```python
from build123d import *

# Parameters (mm, degrees)
F0_R      = 1.75
F0_R_2    = 1.51
F0_R_3    = 1.225
F8_DEPTH  = 0.5
F2_R      = 1.75
F2_R_2    = 1.51
F2_R_3    = 1.225
F9_DEPTH  = 0.5
F7_R      = 1.97
F10_DEPTH = 0.5
F11_DEPTH = 1
F12_DEPTH = 0.5
F13_DEPTH = 25
F16_DEPTH = 0.5
F17_DEPTH = 0.5
F18_W     = 41.976
F18_H     = 1.2
F19_DEPTH = 11.301


# Not quite as in the source:
# - a feature names something its author has since deleted; it is built from what else it names


with BuildPart() as f8:
    # F0 (on Front) → F8 (new body)
    with BuildSketch(Plane.XZ):
        with BuildLine():
            Line((-24.095, 11.6), (-47.125, 11.6))
            Line((-47.125, 11.6), (-47.125, 0))
            Line((-47.125, 0), (47.125, 0))
            ThreePointArc((47.125, 0), (48.3457892371, 4.0785044966), (44.6764603032, 6.2373353065))
            Line((44.6764603032, 6.2373353065), (25.9870177338, 8.0793821146))
            Line((25.9870177338, 8.0793821146), (-19.4229822662, 8.0793821146))
            Line((-19.4229822662, 8.0793821146), (-24.095, 11.6))
        make_face()
        with Locations((-43.275, 3.85)):
            Circle(F0_R, mode=Mode.SUBTRACT)
        with Locations((45.1343327214, 2.8178092836)):
            Circle(F0_R_2, mode=Mode.SUBTRACT)
        with Locations((-40.8, 8.615)):
            Circle(F0_R_3, mode=Mode.SUBTRACT)
    extrude(amount=F8_DEPTH)

    # F6 (on offset) → F9, piece 2 (join)
    with BuildSketch(Plane.YZ.offset(-47.125)):
        Polygon((3.7804580054, 10.7198863682), (3, 11.65), (0, 11.65), (0, 0), (4.5804580054, 0), (4.5804580054, 10.7198863682), align=None)
    extrude(amount=F9_DEPTH)



with BuildPart() as f8b:
    # F2 (on offset) → F8, piece 2 (new body)
    with BuildSketch(Plane.XZ.offset(-10.8)):
        with BuildLine():
            Line((-19.4229822662, 8.0793821146), (-24.095, 11.6))
            Line((-24.095, 11.6), (-47.125, 11.6))
            Line((-47.125, 11.6), (-47.125, 0))
            Line((-47.125, 0), (47.125, 0))
            ThreePointArc((47.125, 0), (48.3457892371, 4.0785044966), (44.6764603032, 6.2373353065))
            Line((44.6764603032, 6.2373353065), (25.9870177338, 8.0793821146))
            Line((25.9870177338, 8.0793821146), (-19.4229822662, 8.0793821146))
        make_face()
        with Locations((-43.275, 3.85)):
            Circle(F2_R, mode=Mode.SUBTRACT)
        with Locations((45.1343327214, 2.8178092836)):
            Circle(F2_R_2, mode=Mode.SUBTRACT)
        with Locations((-40.8, 8.615)):
            Circle(F2_R_3, mode=Mode.SUBTRACT)
    extrude(amount=F8_DEPTH)

    # F6 (on offset) → F9 (join)
    with BuildSketch(Plane.YZ.offset(-47.125)):
        Polygon((10.8, 0), (10.8, 11.65), (7.8, 11.65), (7.0195419946, 10.7198863682), (6.2195419946, 10.7198863682), (6.2195419946, 0), align=None)
    extrude(amount=F9_DEPTH)


with BuildPart() as f8_1:
    add(f8.part)

    add(f8b.part)  # F10 merges F8b
    # F7 (on Top) → F10 (join)
    with BuildSketch(Plane.XY):
        Polygon((-47.125, 4.45), (-47.125, 0), (-46.325, 0), (-46.325, 1.5), (-45.2581904829, 1.5), (-45.2581904829, 9.3), (-46.325, 9.3), (-46.325, 10.8), (-47.125, 10.8), (-47.125, 5.95), align=None)
        Polygon((-46.325, 1.5), (-46.325, 0), (-24.095, 0), (-19.4229822662, 0), (25.9870177338, 0), (44.676, 0), (44.676, 10.8), (25.9870177338, 10.8), (-19.4229822662, 10.8), (-46.325, 10.8), (-46.325, 9.3), (-45.2581904829, 9.3), (-45.2581904829, 1.5), align=None)
        with BuildLine():
            Line((-41.976, 1.89), (-41.976, 8.91))
            ThreePointArc((-41.976, 8.91), (-38.466, 5.4), (-41.976, 1.89))
        make_face(mode=Mode.SUBTRACT)
        with Locations((-29.946, 5.4)):
            Circle(F7_R, mode=Mode.SUBTRACT)
        with Locations((29.946, 5.4)):
            Circle(F7_R, mode=Mode.SUBTRACT)
        with BuildLine():
            Line((41.976, 8.91), (41.976, 1.89))
            ThreePointArc((41.976, 1.89), (38.466, 5.4), (41.976, 8.91))
        make_face(mode=Mode.SUBTRACT)
    extrude(amount=F10_DEPTH)

    # F7 (on Top) → F11 (join)
    with BuildSketch(Plane.XY):
        Polygon((-46.325, 1.5), (-46.325, 0), (-24.095, 0), (-19.4229822662, 0), (25.9870177338, 0), (44.676, 0), (44.676, 10.8), (25.9870177338, 10.8), (-19.4229822662, 10.8), (-46.325, 10.8), (-46.325, 9.3), (-45.2581904829, 9.3), (-45.2581904829, 1.5), align=None)
        with BuildLine():
            Line((-41.976, 1.89), (-41.976, 8.91))
            ThreePointArc((-41.976, 8.91), (-38.466, 5.4), (-41.976, 1.89))
        make_face(mode=Mode.SUBTRACT)
        with Locations((-29.946, 5.4)):
            Circle(F7_R, mode=Mode.SUBTRACT)
        with Locations((29.946, 5.4)):
            Circle(F7_R, mode=Mode.SUBTRACT)
        with BuildLine():
            Line((41.976, 8.91), (41.976, 1.89))
            ThreePointArc((41.976, 1.89), (38.466, 5.4), (41.976, 8.91))
        make_face(mode=Mode.SUBTRACT)
    extrude(amount=F11_DEPTH)

    # F6 (on offset) → F12 (join)
    with BuildSketch(Plane.YZ.offset(-47.125)):
        Polygon((3.7804580054, 10.7198863682), (3, 11.65), (0, 11.65), (0, 0), (4.5804580054, 0), (4.5804580054, 10.7198863682), align=None)
    extrude(amount=F12_DEPTH)

    # F13 (cut): a face of the model
    f13_faces = [f8_1.faces().sort_by_distance(p)[0] for p in [
        (-46.0368491628, 5.3368390391, 0.5),
    ]]
    extrude(f13_faces, amount=-F13_DEPTH, mode=Mode.SUBTRACT)

    # F14 (on face) → F16 (join)
    with BuildSketch(Plane.YZ.offset(-41.976)):
        with BuildLine():
            Line((4, 2.55), (4, 1))
            Line((4, 1), (4.5804580054, 1))
            Line((4.5804580054, 1), (4.5804580054, 1.7362401346))
            ThreePointArc((4.5804580054, 1.7362401346), (4.23, 2.55), (4.5804580054, 3.3637598654))
            Line((4.5804580054, 3.3637598654), (4.5804580054, 3.6591912001))
            ThreePointArc((4.5804580054, 3.6591912001), (4.1538851032, 3.175946606), (4, 2.55))
        make_face()
        with BuildLine():
            ThreePointArc((6.2195419946, 3.5826648631), (5.4129608614, 3.8985310267), (4.5804580054, 3.6591912001))
            Line((4.5804580054, 3.6591912001), (4.5804580054, 3.3637598654))
            ThreePointArc((4.5804580054, 3.3637598654), (5.4235415848, 3.6675829434), (6.2195419946, 3.2559013526))
            Line((6.2195419946, 3.2559013526), (6.2195419946, 3.5826648631))
        make_face()
        with BuildLine():
            Line((4.5804580054, 1.7362401346), (4.5804580054, 1))
            Line((4.5804580054, 1), (6.2195419946, 1))
            Line((6.2195419946, 1), (6.2195419946, 1.8440986474))
            ThreePointArc((6.2195419946, 1.8440986474), (5.4235415848, 1.4324170566), (4.5804580054, 1.7362401346))
        make_face()
        with BuildLine():
            Line((6.2195419946, 1.8440986474), (6.2195419946, 1))
            Line((6.2195419946, 1), (6.7, 1))
            Line((6.7, 1), (6.7, 2.55))
            ThreePointArc((6.7, 2.55), (6.5740060647, 3.1194814779), (6.2195419946, 3.5826648631))
            Line((6.2195419946, 3.5826648631), (6.2195419946, 3.2559013526))
            ThreePointArc((6.2195419946, 3.2559013526), (6.4055299697, 2.9245083217), (6.47, 2.55))
            ThreePointArc((6.47, 2.55), (6.4055299697, 2.1754916783), (6.2195419946, 1.8440986474))
        make_face()
    extrude(amount=-F16_DEPTH)

    # F15 (on face) → F17 (join)
    with BuildSketch(Plane(origin=(41.976, 0, 0), x_dir=(0, -1, 0), z_dir=(-1, 0, 0))):
        with BuildLine():
            ThreePointArc((-4.5804580054, 3.3637598654), (-4.23, 2.55), (-4.5804580054, 1.7362401346))
            Line((-4.5804580054, 1.7362401346), (-4.5804580054, 1))
            Line((-4.5804580054, 1), (-4, 1))
            Line((-4, 1), (-4, 2.55))
            ThreePointArc((-4, 2.55), (-4.1538851032, 3.175946606), (-4.5804580054, 3.6591912001))
            Line((-4.5804580054, 3.6591912001), (-4.5804580054, 3.3637598654))
        make_face()
        with BuildLine():
            Line((-6.2195419946, 3.5826648631), (-6.2195419946, 3.2559013526))
            ThreePointArc((-6.2195419946, 3.2559013526), (-5.4235415848, 3.6675829434), (-4.5804580054, 3.3637598654))
            Line((-4.5804580054, 3.3637598654), (-4.5804580054, 3.6591912001))
            ThreePointArc((-4.5804580054, 3.6591912001), (-5.4129608614, 3.8985310267), (-6.2195419946, 3.5826648631))
        make_face()
        with BuildLine():
            Line((-6.2195419946, 1), (-6.2195419946, 1.8440986474))
            ThreePointArc((-6.2195419946, 1.8440986474), (-6.47, 2.55), (-6.2195419946, 3.2559013526))
            Line((-6.2195419946, 3.2559013526), (-6.2195419946, 3.5826648631))
            ThreePointArc((-6.2195419946, 3.5826648631), (-6.5740060647, 3.1194814779), (-6.7, 2.55))
            Line((-6.7, 2.55), (-6.7, 1))
            Line((-6.7, 1), (-6.2195419946, 1))
        make_face()
        with BuildLine():
            ThreePointArc((-4.5804580054, 1.7362401346), (-5.4235415848, 1.4324170566), (-6.2195419946, 1.8440986474))
            Line((-6.2195419946, 1.8440986474), (-6.2195419946, 1))
            Line((-6.2195419946, 1), (-4.5804580054, 1))
            Line((-4.5804580054, 1), (-4.5804580054, 1.7362401346))
        make_face()
    extrude(amount=-F17_DEPTH)

    # F18 (on face) → F19 (cut, through all)
    with BuildSketch(Plane.XZ.offset(0.5)):
        with Locations((-19.4615396968, 4.8)):
            Rectangle(F18_W, F18_H)
    extrude(amount=-F19_DEPTH, mode=Mode.SUBTRACT)


solid = f8_1.part
```
The listing builds one solid part. Answer for the finished solid, in the listing's coordinates (mm). A direction names the side the tool comes from. Give positions to 0.01 mm unless a question says otherwise; leave off trailing zeros. Loops run counter-clockwise (first coordinate to the right, second up) from the corner with the lowest first, then second, coordinate; pieces in that order, holes last. Notation, with made-up numbers: (-23.5, 83) - (-10.5, 83) arc R27 ccw to (-10.5, 119) - close; hole circle Ø7 at (84.5, 64.5). An arc over 180 degrees is marked (long way). Return JSON: item names as keys, results as strings. Group by question number.
1. Find section B-B (x = 15). Write down the section's boundary in (y, z).
2. Find section A-A (x = -12). Write down the section's boundary in (y, z), then the cut area to 3 significant figures.
3. Given pin 1 Ø5 at (y, z) = (7.5, 9.5) entering from +X (3 decimals); pin 2 Ø6.5 at (x, y) = (-29.946, 5.4) entering from +Z; pin 3 Ø3 at (x, z) = (-43.275, 3.85) entering from -Y, each flat-ended and moving along its own axis, determine where each tip first touches the part or whether it passes through.
4. Find section D-D (x = 40). Write down the section's boundary in (y, z), then the cut area to 3 significant figures.
5. Find section C-C (y = 5.4). State how many separate pieces and enclosed holes the cut face has, then the cut area to 3 significant figures.
6. Determine the mould class of faces 1 (the cylindrical face through (-41.606, -0.246, 4.376)), 2 (the flat face through (35.463, 10.554, 7.145)), 3 (the cylindrical face through (48.37, 10.55, 4.02)) for opening direction Z: pulls with the +Z half, pulls with the -Z half, needs draft (parallel to the pull), parting line crosses it, or undercut.
7. Which of the six approach directions +Z, -Z, +X, -X, +Y, -Y give full straight-line access (tool end or side, diameter ignored) to faces 4 (the flat face through (-42.476, 5.3, 1.2)), 5 (the flat face through (-46.625, 2, 6)), 6 (the flat face through (-21.73, 10.55, 9.82))?
8. Straight lines are drawn through the part: line 1 (Y direction, x = 23, z = 1.25); line 2 (Z direction, x = -40.8, y = -0.05); line 3 (Z direction, x = -30.5, y = 0.5). For each, find the intervals that lie inside material, in ascending order. Write a range as [from, to].
Verdict:
{
 "1": {"outline": "(-0.5, 0) - (10.8, 0) - (10.8, 8.08) - (10.3, 8.08) - (10.3, 1) - (0, 1) - (0, 8.08) - (-0.5, 8.08) - close"},
 "2": {"outline": "(-0.5, 0) - (10.8, 0) - (10.8, 4.2) - (10.3, 4.2) - (10.3, 1) - (0, 1) - (0, 4.2) - (-0.5, 4.2) - close; (-0.5, 5.4) - (0, 5.4) - (0, 8.08) - (-0.5, 8.08) - close; (10.3, 5.4) - (10.8, 5.4) - (10.8, 8.08) - (10.3, 8.08) - close", "area": "17.2 mm^2"},
 "3": {"pin 1": "stops at x = -46.625", "pin 2": "stops at z = 1", "pin 3": "stops at y = 4"},
 "4": {"outline": "(-0.5, 0) - (2.5, 0) - (2.5, 1) - (0, 1) - (0, 6.7) - (-0.5, 6.7) - close; (8.3, 0) - (10.8, 0) - (10.8, 6.7) - (10.3, 6.7) - (10.3, 1) - (8.3, 1) - close", "area": "11.2 mm^2"},
 "5": {"separate pieces": "7", "enclosed holes": "0", "area": "75.7 mm^2"},
 "6": {"face 1": "undercut", "face 2": "pulls with the +Z half", "face 3": "parting line crosses it"},
 "7": {"face 4": "+Z", "face 5": "+Z, -Z", "face 6": "+Z, +X, +Y, -Y"},
 "8": {"line 1": "y = [-0.5, 0], [10.3, 10.8]", "line 2": "z = [0, 7.39], [9.84, 11.6]", "line 3": "z = [0, 1]"}
}
